from build123d import *

# Parameters (mm, degrees)
SKETCH2_R           = 4.1
BOSS_EXTRUDE2_DEPTH = 10


with BuildPart() as part:
    # Sketch2 → Boss-Extrude2 (new body)
    with BuildSketch(Plane.XY):
        with BuildLine():
            ThreePointArc((-8.388352144, 2.232508627), (-7.643352144, 2.753972912), (-8.388352144, 3.275437196))
            Line((-8.388352144, 3.275437196), (-8.388352144, 4.232508627))
            ThreePointArc((-8.388352144, 4.232508627), (-7.805907881, 4.361528648), (-7.67688786, 4.943972912))
            Line((-7.67688786, 4.943972912), (-6.719816429, 4.943972912))
            ThreePointArc((-6.719816429, 4.943972912), (-6.198352144, 4.198972912), (-5.67688786, 4.943972912))
            Line((-5.67688786, 4.943972912), (-4.719816429, 4.943972912))
            ThreePointArc((-4.719816429, 4.943972912), (-4.198352144, 4.198972912), (-3.67688786, 4.943972912))
            Line((-3.67688786, 4.943972912), (-2.719816429, 4.943972912))
            ThreePointArc((-2.719816429, 4.943972912), (-2.198352144, 4.198972912), (-1.67688786, 4.943972912))
            Line((-1.67688786, 4.943972912), (-0.719816429, 4.943972912))
            ThreePointArc((-0.719816429, 4.943972912), (-0.198352144, 4.198972912), (0.32311214, 4.943972912))
            Line((0.32311214, 4.943972912), (1.280183571, 4.943972912))
            ThreePointArc((1.280183571, 4.943972912), (1.409203592, 4.361528648), (1.991647856, 4.232508627))
            Line((1.991647856, 4.232508627), (1.991647856, 3.275437196))
            ThreePointArc((1.991647856, 3.275437196), (1.246647856, 2.753972912), (1.991647856, 2.232508627))
            Line((1.991647856, 2.232508627), (1.991647856, 1.275437196))
            ThreePointArc((1.991647856, 1.275437196), (1.246647856, 0.753972912), (1.991647856, 0.232508627))
            Line((1.991647856, 0.232508627), (1.991647856, -0.724562804))
            ThreePointArc((1.991647856, -0.724562804), (1.246647856, -1.246027088), (1.991647856, -1.767491373))
            Line((1.991647856, -1.767491373), (1.991647856, -2.724562804))
            ThreePointArc((1.991647856, -2.724562804), (1.246647856, -3.246027088), (1.991647856, -3.767491373))
            Line((1.991647856, -3.767491373), (1.991647856, -4.724562804))
            ThreePointArc((1.991647856, -4.724562804), (1.409203592, -4.853582824), (1.280183571, -5.436027088))
            Line((1.280183571, -5.436027088), (0.32311214, -5.436027088))
            ThreePointArc((0.32311214, -5.436027088), (-0.198352144, -4.691027088), (-0.719816429, -5.436027088))
            Line((-0.719816429, -5.436027088), (-1.67688786, -5.436027088))
            ThreePointArc((-1.67688786, -5.436027088), (-2.198352144, -4.691027088), (-2.719816429, -5.436027088))
            Line((-2.719816429, -5.436027088), (-3.67688786, -5.436027088))
            ThreePointArc((-3.67688786, -5.436027088), (-4.198352144, -4.691027088), (-4.719816429, -5.436027088))
            Line((-4.719816429, -5.436027088), (-5.67688786, -5.436027088))
            ThreePointArc((-5.67688786, -5.436027088), (-6.198352144, -4.691027088), (-6.719816429, -5.436027088))
            Line((-6.719816429, -5.436027088), (-7.67688786, -5.436027088))
            ThreePointArc((-7.67688786, -5.436027088), (-7.805907881, -4.853582824), (-8.388352144, -4.724562804))
            Line((-8.388352144, -4.724562804), (-8.388352144, -3.767491373))
            ThreePointArc((-8.388352144, -3.767491373), (-7.643352144, -3.246027088), (-8.388352144, -2.724562804))
            Line((-8.388352144, -2.724562804), (-8.388352144, -1.767491373))
            ThreePointArc((-8.388352144, -1.767491373), (-7.643352144, -1.246027088), (-8.388352144, -0.724562804))
            Line((-8.388352144, -0.724562804), (-8.388352144, 0.232508627))
            ThreePointArc((-8.388352144, 0.232508627), (-7.643352144, 0.753972912), (-8.388352144, 1.275437196))
            Line((-8.388352144, 1.275437196), (-8.388352144, 2.232508627))
        make_face()
        with Locations((-3.198352144, -0.246027088)):
            Circle(SKETCH2_R, mode=Mode.SUBTRACT)
    extrude(amount=BOSS_EXTRUDE2_DEPTH)


solid = part.part
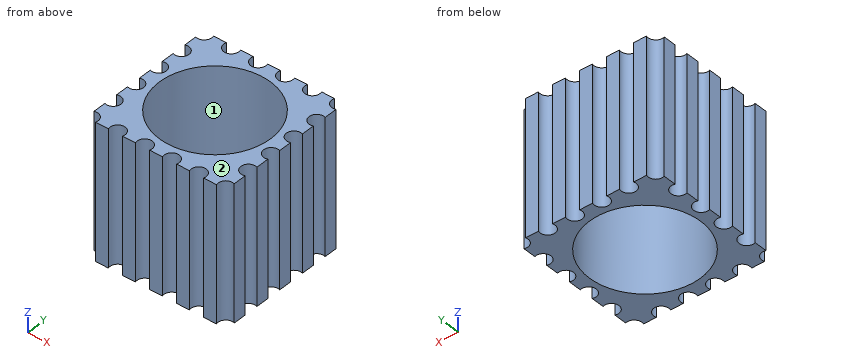
Source: CAD feature listing. Evaluate the final solid. Frame: model axes, mm. Face numbers are marked on the shaded views. Coordinates: 2 decimals unless noted, no trailing zeros. Order: outer loops, then holes, each group sorted by start corner. A loop starts at its lowest first (then second) coordinate and runs counter-clockwise, first axis right, second up. Notation, with made-up numbers: M 47,-12.75 L 51,-12.75 A16 ccw 51,4.25 Z; hole C 38,15 d5. An arc over 180 degrees is marked long. Write each question's results on one line, items separated by ' | '. Start each with the question number.
Item 1: Cut plane B-B (y = 2.75). Return loops of the section in (x, z).
Item 2: Cut plane A-A (x = -6). Return loops of the section in (y, z), and give its area (3 significant figures).
Item 3: First-contact query: pin 1 Ø1.4 at (x, y) = (1.8, -3.25) entering from +Z; pin 2 Ø2 at (x, y) = (-2.5, 2) entering from +Z. Flat tips, straight axial feed; report the tip coordinate or a pass-through.
Item 4: Draft query along Y for the marked faces 1 and 2. Return one class per face: pulls with the +Y half, pulls with the -Y half, needs draft (parallel to the pull), parting line crosses it, or undercut.
Item 5: Line query: probe 1 along Y at (x, z) = (-8, 6); probe 2 along Y at (x, z) = (-3.25, 0.75); probe 3 along Y at (x, z) = (-0.25, 2). Output: solid intervals per line, ascending.
Checked values:
1) outline: M -7.64,0 L -6,0 L -6,10 L -7.64,10 Z; M -0.4,0 L 1.25,0 L 1.25,10 L -0.4,10 Z
2) outline: M -4.73,0 L -3.24,0 L -3.24,10 L -4.73,10 Z; M 2.75,0 L 4.24,0 L 4.24,10 L 2.75,10 Z | area: 29.8 mm2
3) pin 1: stops at z = 10 | pin 2: passes through
4) face 1: undercut | face 2: needs draft
5) probe 1: y = -4.73 to -3.76, -2.73 to -1.76, -0.73 to 0.24, 1.27 to 2.24, 3.27 to 4.24 | probe 2: y = -5.44 to -4.35, 3.85 to 4.94 | probe 3: y = -4.69 to -3.1, 2.6 to 4.2
